from build123d import *

# Parameters (mm, degrees)
SKETCH1_R           = 399
BOSS_EXTRUDE1_DEPTH = 14
SKETCH2_R           = 352
CUT_EXTRUDE1_DEPTH  = 14
SKETCH4_R           = 4
CUT_EXTRUDE2_DEPTH  = 19.304
CIRPATTERN1_COUNT   = 8
SKETCH7_R           = 4
CUT_EXTRUDE3_DEPTH  = 15
CIRPATTERN2_COUNT   = 8


with BuildPart() as part:
    # Sketch1 → Boss-Extrude1 (new body)
    with BuildSketch(Plane(origin=(0, 0, 0), x_dir=(1, 0, 0), z_dir=(0, 1, 0))):
        Circle(SKETCH1_R)
    extrude(amount=BOSS_EXTRUDE1_DEPTH)

    # Sketch2 → Cut-Extrude1 (cut)
    with BuildSketch(Plane(origin=(0, 14, 0), x_dir=(1, 0, 0), z_dir=(0, 1, 0))):
        Circle(SKETCH2_R)
    extrude(amount=-CUT_EXTRUDE1_DEPTH, mode=Mode.SUBTRACT)

    # Sketch4 → Cut-Extrude2 (cut)
    with BuildSketch(Plane(origin=(0, 0, 0), x_dir=(-1, 0, 0), z_dir=(0, -1, 0))):
        with Locations((0, 387.5)):
            Circle(SKETCH4_R)
    cut_extrude2 = extrude(amount=-CUT_EXTRUDE2_DEPTH, mode=Mode.SUBTRACT)

    # CirPattern1: Cut-Extrude2 ×8 about axis
    cirpattern1_axis = Axis((0, 0, 0), (0, 1, 0))
    for i in range(1, CIRPATTERN1_COUNT):
        add(cut_extrude2.rotate(cirpattern1_axis, i * 360 / CIRPATTERN1_COUNT), mode=Mode.SUBTRACT)

    # Sketch7 → Cut-Extrude3 (cut, through all)
    with BuildSketch(Plane(origin=(0, 14, 0), x_dir=(1, 0, 0), z_dir=(0, 1, 0))):
        with Locations((0, 362.5)):
            Circle(SKETCH7_R)
    cut_extrude3 = extrude(amount=-CUT_EXTRUDE3_DEPTH, mode=Mode.SUBTRACT)

    # CirPattern2: Cut-Extrude3 ×8 about axis
    cirpattern2_axis = Axis((0, 0, 0), (0, 1, 0))
    for i in range(1, CIRPATTERN2_COUNT):
        add(cut_extrude3.rotate(cirpattern2_axis, i * 360 / CIRPATTERN2_COUNT), mode=Mode.SUBTRACT)


solid = part.part
Build history of the part. All positions in model axes, mm. Give positions to 0.01 mm unless a question says otherwise; leave off trailing zeros. Order: outer loops, then holes, each group sorted by start corner. A loop starts at its lowest first (then second) coordinate and runs counter-clockwise, first axis right, second up. Notation, with made-up numbers: M 37,-3 L 69,-3 A28 ccw 69,27 Z; hole C 3.5,68.5 d5. An arc over 180 degrees is marked long. Use one line per item in the form item = value.
Q1. Slice it at C-C, the plane y = 6.5. State how many separate pieces and enclosed holes the cut face has, and give its area (3 significant figures).
Conclusion:
separate_pieces = 1
enclosed_holes = 17
area = 110,000 mm2
Q2. Wall check: probe 1 along X at (y, z) = (10, 0); probe 2 along X at (y, z) = (8.75, 114.5). Give the ranges that are in metal, low to high.
Conclusion:
probe_1 = -399 to -391.5, -383.5 to -366.5, -358.5 to -352, 352 to 358.5, 366.5 to 383.5, 391.5 to 399
probe_2 = -382.22 to -332.86, 332.86 to 382.22
Q3. Slice it at A-A, the plane z = -186. Write the cut outline in (x, y), and give its area (3 significant figures).
Conclusion:
outline = M -352.99,0 L -298.84,0 L -298.84,14 L -352.99,14 Z; M 298.84,0 L 352.99,0 L 352.99,14 L 298.84,14 Z
area = 1,520 mm2
Q4. Pull direction X, two halves, no side cores. Call faces 1 (the cylindrical face through (380.575, 6.902, -119.849)), 2 (the flat face through (235, 0, -268)), 3 (the cylindrical face through (-76.31, 7.1, 343.63)): released by +X, released by -X, zero draft, split by the parting line, or undercut.
Conclusion:
face_1 = split by the parting line
face_2 = zero draft
face_3 = undercut
Q5. Slice it at B-B, the plane x = 167.5. Write the cut outline in (y, z).
Conclusion:
outline = M 0,-362.14 L 14,-362.14 L 14,-309.59 L 0,-309.59 Z; M 0,309.59 L 14,309.59 L 14,362.14 L 0,362.14 Z
Q6. Pin check, flat tips, straight feed: P1, Ø3, axis at y = 6, z = 197.5, coming from the -X side; P2, Ø4, axis at y = 8.5, z = -279.5, coming from the -X side; P3, Ø5, axis at x = 274, z = 274, coming from the +Y side; P4, Ø6, axis at y = 9, z = 271, coming from the -X side. Stop position of each tip, or through.
Conclusion:
P1 = -347.54
P2 = -286.7
P3 = through
P4 = -295.6
